Can you work these out from the drawing? Everything is in mm from the part's minimum corner. A direction names the side the tool comes from. Coordinates: 2 decimals unless noted, no trailing zeros. Loops run counter-clockwise (first coordinate to the right, second up) from the corner with the lowest first, then second, coordinate; pieces in that order, holes last. Notation, with made-up numbers: (-2.5, -4.5) - (47.5, -4.5) arc R30 cw to (47.5, 20.5) - close; hole circle Ø11 at (16.5, 0). An arc over 180 degrees is marked (long way). Put each result on its own line as item: value. Start each with the question number.
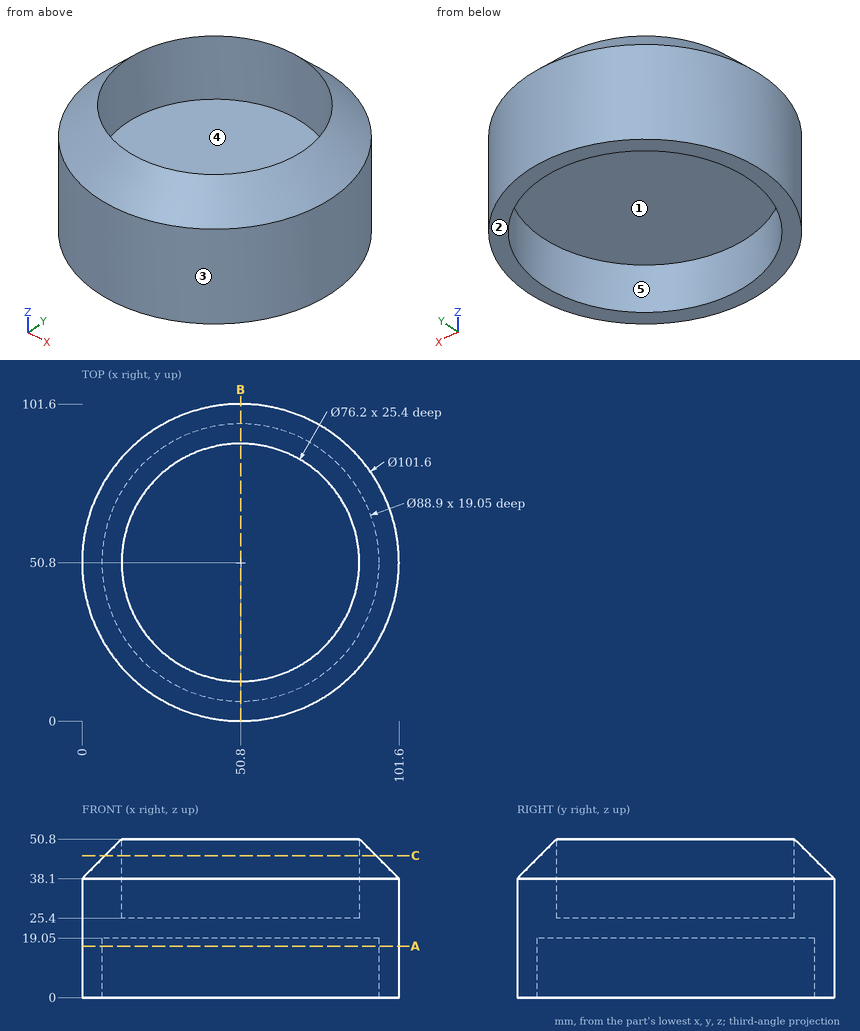
(1) If we mould it in two halves opening along X, with no side actions, what happens to the marked faces 1, 2 and 3? For each: pulls with the +X half, pulls with the -X half, needs draft (parallel to the pull), parting line crosses it, or undercut.
(2) I want a section at A-A on z = 16.5. List the corners of the cut face in (x, y) for me, and give its area (3 significant figures).
(3) I want a section at B-B on x = 50.8. List the corners of the cut face in (y, z) for me, and give its area (3 significant figures).
(4) Which directions (+Z, -Z, +X, -X, +Y, -Y) give clear straight access to the entire face, cutting with the end or side of a thin tool? Please do the marked faces 4 and 5.
(5) I need wall thicknesses on L1, parallel to Y at x = 50.8, z = 5.25; L2, parallel to Y at x = 50, z = 36; L3, parallel to X at y = 50, z = 11. Which ranges of each line are inside material? Lowest first, please. Write a range as [from, to].
(6) For pin 1 Ø2 at (y, z) = (79.5, 28.5) entering from -X; pin 2 Ø3 at (x, z) = (11.5, 10.5) entering from +Y; pin 3 Ø8 at (x, y) = (74, 30.5) entering from -Z, each with a flat end and sliding along its axis, tell me the tip position at first contact or that it passes through.
(7) I want a section at C-C on z = 45.5. List the corners of the cut face in (x, y) for me.
Answer sheet:
1. face 1: undercut
1. face 2: needs draft
1. face 3: parting line crosses it
2. outline: circle Ø101.6 at (50.8, 50.8); hole circle Ø88.9 at (50.8, 50.8)
2. area: 1,900 mm^2
3. outline: (0, 0) - (6.35, 0) - (6.35, 19.05) - (95.25, 19.05) - (95.25, 0) - (101.6, 0) - (101.6, 38.1) - (88.9, 50.8) - (88.9, 25.4) - (12.7, 25.4) - (12.7, 50.8) - (0, 38.1) - close
3. area: 1,370 mm^2
4. face 4: +Z
4. face 5: -Z
5. L1: y = [0, 6.35], [95.25, 101.6]
5. L2: y = [0.01, 12.71], [88.89, 101.59]
5. L3: x = [0.01, 6.36], [95.24, 101.59]
6. pin 1: stops at x = 8.22
6. pin 2: stops at y = 84.74
6. pin 3: stops at z = 19.05
7. outline: circle Ø86.8 at (50.8, 50.8); hole circle Ø76.2 at (50.8, 50.8)
